```python
from build123d import *

# Parameters (mm, degrees)
CROQUIS1_W              = 400
CROQUIS1_H              = 600
SALIENTE_EXTRUIR1_DEPTH = 30
CROQUIS3_W              = 320
CROQUIS3_H              = 20
SALIENTE_EXTRUIR2_DEPTH = 735
CROQUIS4_W              = 50
CROQUIS4_H              = 695
CORTAR_EXTRUIR1_DEPTH   = 550.471728
CROQUIS5_W              = 20
CROQUIS5_H              = 20
SALIENTE_EXTRUIR3_DEPTH = 458.943456


with BuildPart() as part:
    # Croquis1 → Saliente-Extruir1 (new body)
    with BuildSketch(Plane.XY):
        Rectangle(CROQUIS1_W, CROQUIS1_H)
    extrude(amount=SALIENTE_EXTRUIR1_DEPTH)

    # Croquis3 → Saliente-Extruir2 (add)
    with BuildSketch(Plane(origin=(0, 0, 0), x_dir=(-1, 0, 0), z_dir=(0, 0, -1))):
        with Locations((0, 239.471728)):
            Rectangle(CROQUIS3_W, CROQUIS3_H)
    saliente_extruir2 = extrude(amount=SALIENTE_EXTRUIR2_DEPTH)

    # Simetría1: Saliente-Extruir2 across plane
    add(saliente_extruir2.mirror(Plane.ZX))

    # Croquis4 → Cortar-Extruir1 (cut, through all)
    with BuildSketch(Plane.XZ.offset(249.471728)):
        with Locations((-135, -367.5)):
            Rectangle(CROQUIS4_W, CROQUIS4_H)
        with Locations((135, -367.5)):
            Rectangle(CROQUIS4_W, CROQUIS4_H)
    extrude(amount=-CORTAR_EXTRUIR1_DEPTH, mode=Mode.SUBTRACT)

    # Croquis5 → Saliente-Extruir3 (add)
    with BuildSketch(Plane.XZ.offset(-229.471728)):
        with Locations((-100, -210)):
            Rectangle(CROQUIS5_W, CROQUIS5_H)
    saliente_extruir3 = extrude(amount=SALIENTE_EXTRUIR3_DEPTH)

    # Simetría2: Saliente-Extruir3 across plane
    add(saliente_extruir3.mirror(Plane(origin=(0, 0, 0), x_dir=(0, 0, 1), z_dir=(1, 0, 0))))


solid = part.part
```
Could you check a few things on this model? Use its own coordinates, in mm. A direction names the side the tool comes from. Give positions to 0.01 mm unless a question says otherwise; leave off trailing zeros. Loops run counter-clockwise (first coordinate to the right, second up) from the corner with the lowest first, then second, coordinate; pieces in that order, holes last. Notation, with made-up numbers: (22, 39.25) - (73, 39.25) arc R27 ccw to (73, 70.25) - close; hole circle Ø10 at (-37.5, -3). An arc over 180 degrees is marked (long way). Use one line per item in the form item = value.
1. I want a section at D-D (x = 70). Please give me the cut outline in (y, z).
Response values:
outline = (-300, 0) - (-249.47, 0) - (-249.47, -735) - (-229.47, -735) - (-229.47, 0) - (229.47, 0) - (229.47, -735) - (249.47, -735) - (249.47, 0) - (300, 0) - (300, 30) - (-300, 30) - close
2. I'm going to push flat-ended pins straight in: pin 1 Ø2 at (x, y) = (-43, 185.5) entering from -Z; pin 2 Ø5 at (x, z) = (-48.5, -574) entering from +Y; pin 3 Ø22 at (y, z) = (241.5, -5.5) entering from +X; pin 4 Ø16 at (y, z) = (239.5, -721) entering from +X. Where does each tip first touch, or does it pass through?
Response values:
pin_1 = 0
pin_2 = 249.47
pin_3 = 200
pin_4 = 160
3. I want a section at C-C (x = -135.5). Please give me the cut outline in (y, z).
Response values:
outline = (-300, 0) - (-249.47, 0) - (-249.47, -20) - (-229.47, -20) - (-229.47, 0) - (229.47, 0) - (229.47, -20) - (249.47, -20) - (249.47, 0) - (300, 0) - (300, 30) - (-300, 30) - close; (-249.47, -735) - (-229.47, -735) - (-229.47, -715) - (-249.47, -715) - close; (229.47, -735) - (249.47, -735) - (249.47, -715) - (229.47, -715) - close
4. I need wall thicknesses on probe 1 along Y at (x, z) = (52, -130); probe 2 along Z at (x, y) = (116.5, 243); probe 3 along Z at (x, y) = (178, -187). Which ranges of each line are inside material? Lowest first, please.
Response values:
probe_1 = -249.47 to -229.47, 229.47 to 249.47
probe_2 = -735 to -715, -20 to 30
probe_3 = 0 to 30
5. Thinking about a two-plate mould opening in Z: for faces 6 (the face through (-135, 239, -715)), 7 (the face through (-160, -239, -725)), 8 (the face through (2, 240, -735)), which applies, released by +Z, released by -Z, zero draft, split by the parting line, or undercut?
Response values:
face_6 = undercut
face_7 = zero draft
face_8 = released by -Z
6. On a 3-axis mill with a long thin cutter (end or side, diameter ignored), from which of +Z, -Z, +X, -X, +Y, -Y can I reach the whole of each face in a straight line? I mean faces 1 (the face through (2, 249.472, -362)), 2 (the face through (-160, -239, -10)), 3 (the face through (-135, -240, -715)), 4 (the face through (100, 3, -200)), 5 (the face through (160, -239, -725)). Say none if no direction works.
Response values:
face_1 = -Z, +X, -X, +Y
face_2 = -Z, -X, +Y, -Y
face_3 = -X, +Y, -Y
face_4 = +X, -X
face_5 = -Z, +X, +Y, -Y
7. I want a section at B-B (y = -95). Please give me the cut outline in (x, z), and give its area (3 significant figures).
Response values:
outline = (-200, 0) - (200, 0) - (200, 30) - (-200, 30) - close; (-110, -220) - (-90, -220) - (-90, -200) - (-110, -200) - close; (90, -220) - (110, -220) - (110, -200) - (90, -200) - close
area = 12,800 mm²
8. I want a section at A-A (z = -111.5). Please give me the cut outline in (x, y), and give its area (3 significant figures).
Response values:
outline = (-110, -249.47) - (110, -249.47) - (110, -229.47) - (-110, -229.47) - close; (-110, 229.47) - (110, 229.47) - (110, 249.47) - (-110, 249.47) - close
area = 8,800 mm²
